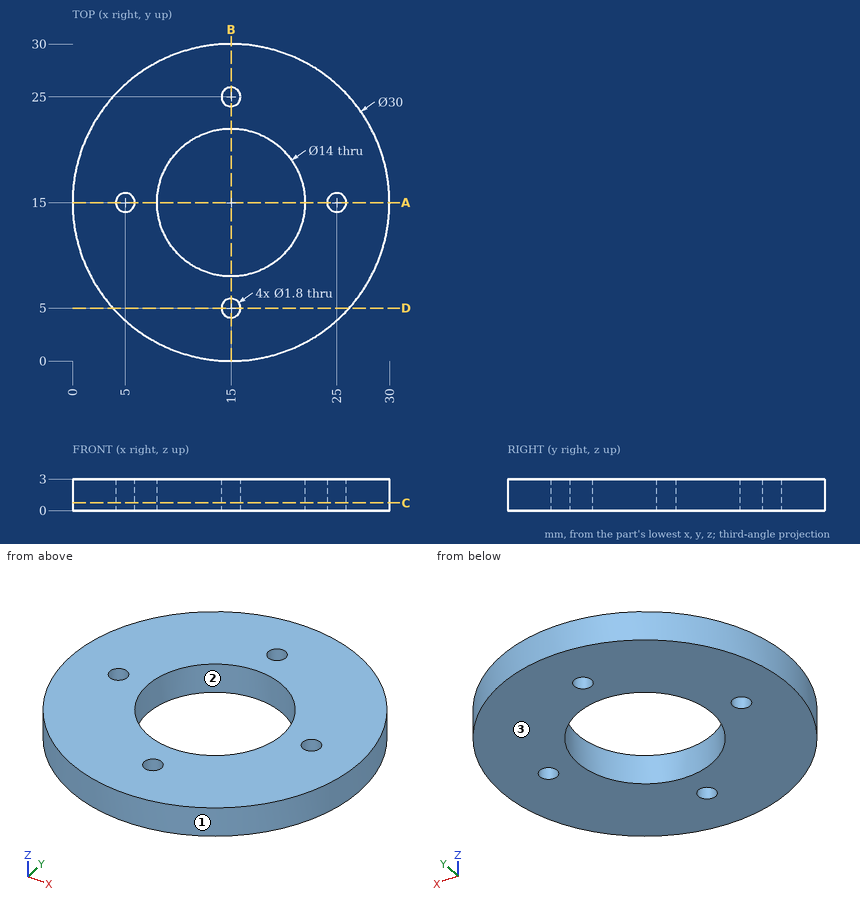
The drawing under review shows one solid part. Ordinate dimensions are in mm from its lowest x, y, z. Round coordinates to 2 decimals unless told otherwise and drop trailing zeros. Write each loop counter-clockwise with the first axis right and the second up, starting at its lowest first coordinate (ties: lowest second). Pieces come first, ordered by that corner, then holes. Notation, with made-up numbers: (49.5, 53) - (59.5, 53) arc R15 ccw to (59.5, 82) - close; hole circle Ø3 at (72.5, -3.5). An arc over 180 degrees is marked (long way). Use one line per item in the form item = value.
Q1. Draft analysis for pull direction Y (two halves, no side actions). For the marked faces 1, 2 and 3, state which applies: +Y half, -Y half, draft (parallel to the pull), parting line (faces both ways), or undercut.
Answer key:
face_1 = parting line
face_2 = undercut
face_3 = draft
Q2. Consider section A-A (y = 15). State the section outline as (x, z) points.
Answer key:
outline = (0, 0) - (4.1, 0) - (4.1, 3) - (0, 3) - close; (5.9, 0) - (8, 0) - (8, 3) - (5.9, 3) - close; (22, 0) - (24.1, 0) - (24.1, 3) - (22, 3) - close; (25.9, 0) - (30, 0) - (30, 3) - (25.9, 3) - close
Q3. Consider section D-D (y = 5). State the section outline as (x, z) points.
Answer key:
outline = (3.82, 0) - (14.1, 0) - (14.1, 3) - (3.82, 3) - close; (15.9, 0) - (26.18, 0) - (26.18, 3) - (15.9, 3) - close
Q4. For line 1 (Y direction, x = 15, z = 1.6); line 2 (Y direction, x = 5, z = 1.9); line 3 (Y direction, x = 24.5, z = 0.6), list the stretches that pass through material, from the lowest coordinate up. Write a range as [from, to].
Answer key:
line_1 = [0, 4.1], [5.9, 8], [22, 24.1], [25.9, 30]
line_2 = [3.82, 14.1], [15.9, 26.18]
line_3 = [3.39, 14.25], [15.75, 26.61]
Q5. Consider section C-C (z = 0.75). State the section outline as (x, y) points.
Answer key:
outline = circle Ø30 at (15, 15); hole circle Ø1.8 at (5, 15); hole circle Ø14 at (15, 15); hole circle Ø1.8 at (15, 5); hole circle Ø1.8 at (15, 25); hole circle Ø1.8 at (25, 15)
Q6. Insertion check: pin 1 Ø1 at (x, z) = (4, 1.5) entering from -Y; pin 2 Ø11 at (x, y) = (15, 15) entering from +Z; pin 3 Ø1 at (y, z) = (10.5, 1) entering from -X. Each pin has a flat end and moves straight along its axis. Give the tip position at first contact, or say it passes through.
Answer key:
pin_1 = 4.29
pin_2 = through
pin_3 = 0.54
